Can you work these out from the model? Positions are in its coordinate system, mm. Face numbers are marked on the shaded views. A direction names the side the tool comes from. Coordinates: 2 decimals unless noted, no trailing zeros. Loops run counter-clockwise (first coordinate to the right, second up) from the corner with the lowest first, then second, coordinate; pieces in that order, holes last. Notation, with made-up numbers: (35, 46.25) -> (71, 46.25) arc R37 cw to (71, 83.25) -> close; hole circle Ø7 at (87, 64.25). An arc over 180 degrees is marked (long way). Use one line per item in the form item = value. Start each with the question number.
(1) Imagine slicing it at C-C (z = 25.4). List the corners of the cut face in (x, y) for me.
(2) On a 3-axis mill with a long thin cutter (end or side, diameter ignored), from which of +Z, -Z, +X, -X, +Y, -Y can I reach the whole of each face in a straight line? I mean the marked faces 1, 2 and 3. Say none if no direction works.
(3) Imagine slicing it at A-A (y = 19). List the corners of the cut face in (x, z) for me.
(4) Imagine slicing it at B-B (x = 88.9). List the corners of the cut face in (y, z) for me, plus the area to 3 significant figures.
(5) I need wall thicknesses on line 1 (X direction, y = 38.1, z = 8.25); line 2 (Z direction, x = 93, y = 19); line 3 (Y direction, x = 91, z = 26.5). Which ranges of each line are inside material? Lowest first, please. Write a range as [from, to].
(6) I'm going to push flat-ended pins straight in: pin 1 (10 mm diameter, centred on y = 55.5, z = 16, fed in from -X); pin 2 (2 mm diameter, centred on y = 11, z = 25, fed in from -X); pin 3 (15 mm diameter, centred on x = 88.9, y = 38.1, fed in from -Z); pin 4 (5 mm diameter, centred on y = 26.5, z = 8, fed in from -X). Where does each tip first touch, or does it pass through?
(7) Imagine slicing it at D-D (z = 45.5). List the corners of the cut face in (x, y) for me.
(8) Thinking about a two-plate mould opening in X: for the marked faces 4, 5, 6 and 7, which applies, released by +X, released by -X, zero draft, split by the parting line, or undercut?
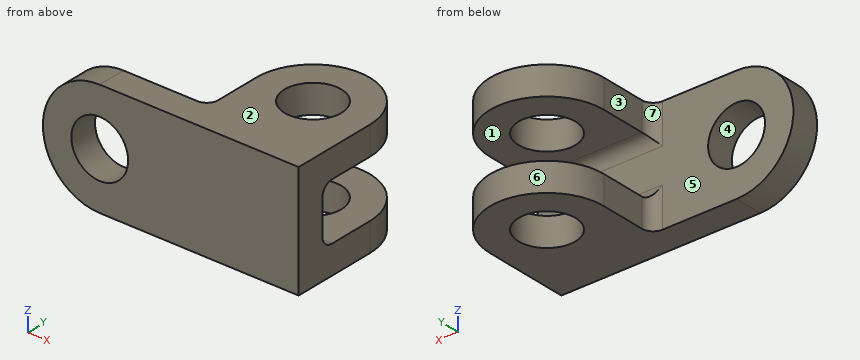
Autodesk Fusion 360 part; units mm, degrees
sketch "Sketch5" plane through (0, 0, 0) normal (0, 0, 1) x (1, 0, 0)
  line L0 (0, 0) -> (114.3, 0)
  line L1 (114.3, 0) -> (114.3, 38.1)
  line L2 (114.3, 63.5) -> (104.14, 63.5)
  line L3 (0, 12.7) -> (0, 0)
  circle A0 centre (88.9, 38.1) radius 12.7
  arc A1 (114.3, 38.1) -> (63.5, 38.1) centre (88.9, 38.1) ccw
  line L4 (63.5, 38.1) -> (63.5, 12.7)
  line L5 (63.5, 12.7) -> (60.96, 12.7)
  line L6 (60.96, 12.7) -> (0, 12.7)
  dimension "d17" = 114.3
  dimension "d18" = 63.5
  dimension "d19" = 25.4
  dimension "d21" = 25.4
  dimension "d22" = 25.4
extrude "Extrude4" add sketch "Sketch5" along normal blind 50.8
sketch "Sketch6" plane through (0, 12.7, 0) normal (0, 1, 0) x (-1, 0, 0)
  line L0 (-63.5, 0) -> (0, 0)
  line L1 (0, 0) -> (0, 50.8)
  line L2 (0, 50.8) -> (-63.5, 50.8)
  line L3 (-63.5, 50.8) -> (-63.5, 0)
  circle A0 centre (-25.4, 25.4) radius 12.7
  arc A1 (-25.4, 0) -> (-25.4, 50.8) centre (-25.4, 25.4) ccw
  dimension "d25" = 25.4
extrude "Extrude5" cut sketch "Sketch6" against normal blind 15.24 contours L0 L1 A1 | L1 L2 A1 | A0
sketch "Sketch7" plane through (63.5, 0, 0) normal (-1, 0, 0) x (0, 0, 1)
  line L0 (0, 38.1) -> (0, 12.7)
  line L1 (0, 12.7) -> (50.8, 12.7)
  line L2 (50.8, 12.7) -> (50.8, 38.1)
  line L3 (50.8, 38.1) -> (0, 38.1)
  line L4 (12.7, 63.5) -> (38.1, 63.5)
  line L5 (38.1, 63.5) -> (38.1, 12.7)
  line L6 (38.1, 12.7) -> (12.7, 12.7)
  line L7 (12.7, 12.7) -> (12.7, 63.5)
extrude "Extrude6" cut sketch "Sketch7" against normal blind 60.96 contours L3 L4 L5 L7 | L1 L3 L5 L6 L7
fillet "Fillet1" radius 5.08 1 edges at (63.5, 12.7, 44.45)
fillet "Fillet2" radius 5.08 1 edges at (63.5, 12.7, 6.35)
fillet "Fillet3" radius 5.08 1 edges at (86.36, 12.7, 12.7)
fillet "Fillet4" radius 5.08 1 edges at (86.36, 12.7, 38.1)
Worked out:
q1.outline = (0, 0) -> (12.7, 0) -> (12.7, 12.7) -> (0, 12.7) -> close; (38.1, 0) -> (114.3, 0) -> (114.3, 12.7) -> (38.1, 12.7) -> close
q2.face_1 = +X, -X, +Y
q2.face_2 = +Z, +X, -X, +Y, -Y
q2.face_3 = +Z, -Z, -X, +Y
q3.outline = (63.5, 0) -> (114.3, 0) -> (114.3, 12.7) -> (63.5, 12.7) -> close; (63.5, 38.1) -> (114.3, 38.1) -> (114.3, 50.8) -> (63.5, 50.8) -> close
q4.outline = (0, 0) -> (25.4, 0) -> (25.4, 12.7) -> (17.78, 12.7) arc R5.08 cw to (12.7, 17.78) -> (12.7, 33.02) arc R5.08 cw to (17.78, 38.1) -> (25.4, 38.1) -> (25.4, 50.8) -> (0, 50.8) -> close; (50.8, 0) -> (63.5, 0) -> (63.5, 12.7) -> (50.8, 12.7) -> close; (50.8, 38.1) -> (63.5, 38.1) -> (63.5, 50.8) -> (50.8, 50.8) -> close
q4.area = 1,300 mm2
q5.line_1 = [63.5, 76.2], [101.6, 114.3]
q5.line_2 = [0, 12.7], [38.1, 50.8]
q5.line_3 = [0, 12.7]
q6.pin_1 = 67.48
q6.pin_2 = 0
q6.pin_3 = through
q6.pin_4 = 63.5
q7.outline = (9.87, 0) -> (114.3, 0) -> (114.3, 38.1) arc R25.4 ccw to (63.5, 38.1) -> (63.5, 17.78) arc R5.08 cw to (58.42, 12.7) -> (9.87, 12.7) -> close; hole circle Ø25.4 at (88.9, 38.1)
q8.face_4 = undercut
q8.face_5 = zero draft
q8.face_6 = split by the parting line
q8.face_7 = released by -X
